The model under review builds one solid part; all positions refer to its coordinate system, in mm. Face numbers are marked on the shaded views. Round coordinates to 2 decimals unless told otherwise and drop trailing zeros. Order: outer loops, then holes, each group sorted by start corner. A loop starts at its lowest first (then second) coordinate and runs counter-clockwise, first axis right, second up. Notation, with made-up numbers: (74.5, 53) - (80.5, 53) arc R16 ccw to (80.5, 81) - close; hole circle Ø1 at (85, 56). An arc over 180 degrees is marked (long way). One line per question, with ' | ' between items. Start each with the question number.
Item 1: Add section A-A on x = 0. State the section outline as (y, z) points (3 decimals).
Item 2: Add section C-C on z = 0. State the section outline as (x, y) points (3 decimals).
Item 3: Insertion check: pin 1 Ø1.5 at (x, y) = (-9.5, 58) entering from +Z; pin 2 Ø7.5 at (x, z) = (49, -12.5) entering from +Y; pin 3 Ø6 at (y, z) = (58, 15.5) entering from -X. Each pin has a flat end and moves straight along its axis. Give the tip position at first contact, or say it passes through.
Item 4: Add section B-B on z = 25.5. State the section outline as (x, y) points, and give its area (3 significant figures).
Item 5: Add section D-D on x = 37. State the section outline as (y, z) points.
Item 6: For L1, parallel to X at y = 6.75, z = 0; L2, parallel to Z at x = 0, y = 63.25; L3, parallel to Y at x = 0, z = 10, list the stretches that pass through material, from the lowest coordinate up. Write a range as [from, to].
Item 7: Draft analysis for pull direction Z (two halves, no side actions). For the marked faces 1, 2, 3 and 4, state which applies: +Z half, -Z half, draft (parallel to the pull), parting line (faces both ways), or undercut.
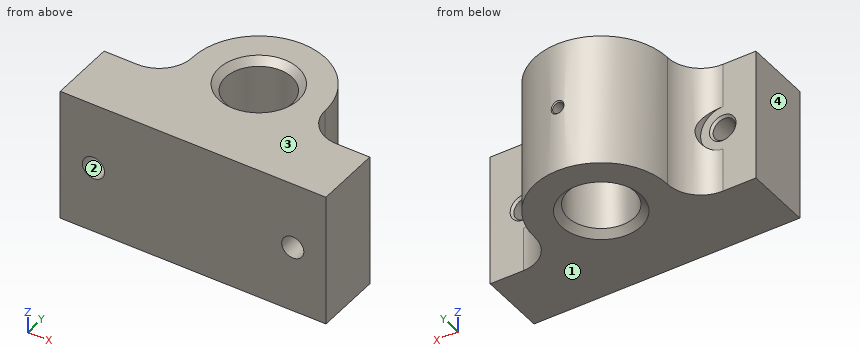
from build123d import *

# Parameters (mm, degrees)
SKETCH1_W                   = 120
SKETCH1_H                   = 60
BOSS_EXTRUDE1_DEPTH         = 30
SKETCH2_R                   = 30
BOSS_EXTRUDE2_DEPTH         = 60
SKETCH3_R                   = 15
CUT_EXTRUDE1_DEPTH          = 114.247516529
CHAMFER1_SIZE               = 3
FILLET2_R                   = 15
SKETCH4_R                   = 10
CUT_EXTRUDE2_DEPTH          = 5
SKETCH5_R                   = 5
CUT_EXTRUDE3_DEPTH          = 81.777472144
CHAMFER2_SIZE               = 1
M6_TAPPED_HOLE2_D           = 5
M6_TAPPED_HOLE2_DEPTH       = 29.999
M6_TAPPED_HOLE2_CSINK_D     = 6.05
M6_TAPPED_HOLE2_CSINK_ANGLE = 90
M6_TAPPED_HOLE2_TIP         = 1.502151548


with BuildPart() as part:
    # Sketch1 → Boss-Extrude1 (new body)
    with BuildSketch(Plane(origin=(0, 0, 0), x_dir=(1, 0, 0), z_dir=(0, 1, 0))):
        Rectangle(SKETCH1_W, SKETCH1_H)
    extrude(amount=BOSS_EXTRUDE1_DEPTH)

    # Sketch2 → Boss-Extrude2 (add)
    with BuildSketch(Plane.XY.offset(30)):
        with Locations((0, 45)):
            Circle(SKETCH2_R)
    extrude(amount=-BOSS_EXTRUDE2_DEPTH)

    # Sketch3 → Cut-Extrude1 (cut, through all)
    with BuildSketch(Plane.XY.offset(30)):
        with Locations((0, 45)):
            Circle(SKETCH3_R)
    extrude(amount=-CUT_EXTRUDE1_DEPTH, mode=Mode.SUBTRACT)

    # Chamfer1
    chamfer1_edges = [part.edges().sort_by_distance(p)[0] for p in [
        (-15, 45, -30),
        (-15, 45, 30),
    ]]
    chamfer(chamfer1_edges, length=CHAMFER1_SIZE)

    # Fillet2
    fillet2_edges = [part.edges().sort_by_distance(p)[0] for p in [
        (-25.980762114, 30, 0),
        (25.980762114, 30, 0),
    ]]
    fillet(fillet2_edges, radius=FILLET2_R)

    # Sketch4 → Cut-Extrude2 (cut)
    with BuildSketch(Plane(origin=(0, 30, 0), x_dir=(1, 0, 0), z_dir=(0, 1, 0))):
        with Locations((-45, 0)):
            Circle(SKETCH4_R)
        with Locations((45, 0)):
            Circle(SKETCH4_R)
    extrude(amount=CUT_EXTRUDE2_DEPTH, mode=Mode.SUBTRACT)

    # Sketch5 → Cut-Extrude3 (cut, through all)
    with BuildSketch(Plane(origin=(0, 30, 0), x_dir=(1, 0, 0), z_dir=(0, 1, 0))):
        with Locations(Location((-45, 0, 0), (0, 0, 270))):
            Circle(SKETCH5_R)
        with Locations(Location((45, 0, 0), (0, 0, 270))):
            Circle(SKETCH5_R)
    extrude(amount=-CUT_EXTRUDE3_DEPTH, mode=Mode.SUBTRACT)

    # Chamfer2
    chamfer2_edges = [part.edges().sort_by_distance(p)[0] for p in [
        (-45, 30, -5),
        (45, 30, -5),
    ]]
    chamfer(chamfer2_edges, length=CHAMFER2_SIZE)

    # M6 Tapped Hole2
    with Locations(Plane(origin=(0, 75, 0), x_dir=(1, 0, 0), z_dir=(0, 1, 0))):
        with Locations((0, 0)):
            CounterSinkHole(M6_TAPPED_HOLE2_D / 2, M6_TAPPED_HOLE2_CSINK_D / 2, depth=M6_TAPPED_HOLE2_DEPTH, counter_sink_angle=M6_TAPPED_HOLE2_CSINK_ANGLE)
            with Locations((0, 0, -(M6_TAPPED_HOLE2_DEPTH + M6_TAPPED_HOLE2_TIP / 2))):  # 118° drill point
                Cone(0, M6_TAPPED_HOLE2_D / 2, M6_TAPPED_HOLE2_TIP, mode=Mode.SUBTRACT)


solid = part.part
Determined:
1) outline: (0, -30) - (27, -30) - (30, -27) - (30, 27) - (27, 30) - (0, 30) - close; (60, -27) - (63, -30) - (75, -30) - (75, -3.025) - (74.475, -2.5) - (60, -2.5) - close; (60, 2.5) - (74.475, 2.5) - (75, 3.025) - (75, 30) - (63, 30) - (60, 27) - close
2) outline: (-60, 0) - (-50, 0) - (-50, 29) - (-51, 30) - (-60, 30) - close; (-40, 0) - (40, 0) - (40, 29) - (39, 30) - (35, 30) - (35, 33.82) arc R15 cw to (30, 45) arc R30 ccw to (2.886, 74.861) - (2.5, 74.475) - (2.5, 59.79) arc R15 cw (long way) to (-2.5, 59.79) - (-2.5, 74.475) - (-2.886, 74.861) arc R30 ccw to (-30, 45) arc R15 cw to (-35, 33.82) - (-35, 30) - (-39, 30) - (-40, 29) - close; (50, 0) - (60, 0) - (60, 30) - (51, 30) - (50, 29) - close
3) pin 1: z = 28.85 | pin 2: y = 30 | pin 3: x = -28.28
4) outline: (-60, 0) - (60, 0) - (60, 30) - (45, 30) arc R15 cw to (30, 45) arc R30 ccw to (-30, 45) arc R15 cw to (-45, 30) - (-60, 30) - close; hole circle Ø30 at (0, 45) | area: 5,300 mm2
5) outline: (0, -30) - (32.31, -30) - (32.31, -6) - (30, -6) - (30, 6) - (32.31, 6) - (32.31, 30) - (0, 30) - close
6) L1: [-60, -50], [-40, 40], [50, 60] | L2: [-30, -2.5], [2.5, 30] | L3: [0, 30], [60, 75]
7) face 1: -Z half | face 2: undercut | face 3: +Z half | face 4: draft
